The listing builds one solid part. Answer for the finished solid, in the listing's coordinates (mm). Give positions to 0.01 mm unless a question says otherwise; leave off trailing zeros. Write each loop counter-clockwise with the first axis right and the second up, starting at its lowest first coordinate (ties: lowest second). Pieces come first, ordered by that corner, then holes. Notation, with made-up numbers: M 71.5,-16 L 118.5,-16 A11 cw 118.5,3 Z; hole C -31.5,30.5 d11. An arc over 180 degrees is marked long. Answer as a JSON object with one key per item and string values.
```python
from build123d import *

# Parameters (mm, degrees)
SKETCH_1_R          = 1.5
SKETCH_1_W          = 4
SKETCH_1_H          = 35
EXTRUDE_1_DEPTH     = 3
FILLET_1_R          = 2
SKETCH_2_R          = 11
CUT_EXTRUDE_1_DEPTH = 3


with BuildPart() as part:
    # 草图1 → 凸台-拉伸1 (new body)
    with BuildSketch(Plane.XY):
        Polygon((-20, 25), (-25, 20), (-25, -75), (-20, -80), (20, -80), (25, -75), (25, 20), (20, 25), align=None)
        with Locations((-15.5, 15.5)):
            Circle(SKETCH_1_R, mode=Mode.SUBTRACT)
        with Locations((15.5, 15.5)):
            Circle(SKETCH_1_R, mode=Mode.SUBTRACT)
        with Locations((15.5, -15.5)):
            Circle(SKETCH_1_R, mode=Mode.SUBTRACT)
        with Locations((-15.5, -15.5)):
            Circle(SKETCH_1_R, mode=Mode.SUBTRACT)
        with Locations((-15.5, -55)):
            Rectangle(SKETCH_1_W, SKETCH_1_H, mode=Mode.SUBTRACT)
        with Locations((15.5, -55)):
            Rectangle(SKETCH_1_W, SKETCH_1_H, mode=Mode.SUBTRACT)
    extrude(amount=EXTRUDE_1_DEPTH)

    # 圆角1
    fillet_1_edges = [part.edges().sort_by_distance(p)[0] for p in [
        (17.5, -72.5, 1.5),
        (-13.5, -72.5, 1.5),
        (13.5, -37.5, 1.5),
        (-17.5, -37.5, 1.5),
        (-17.5, -72.5, 1.5),
        (13.5, -72.5, 1.5),
        (17.5, -37.5, 1.5),
        (-13.5, -37.5, 1.5),
    ]]
    fillet(fillet_1_edges, radius=FILLET_1_R - 0.0001)  # a hair under: the kernel refuses the full size

    # 草图2 → 切除-拉伸1 (cut)
    with BuildSketch(Plane.XY.offset(3)):
        Circle(SKETCH_2_R)
    extrude(amount=-CUT_EXTRUDE_1_DEPTH, mode=Mode.SUBTRACT)


solid = part.part
```
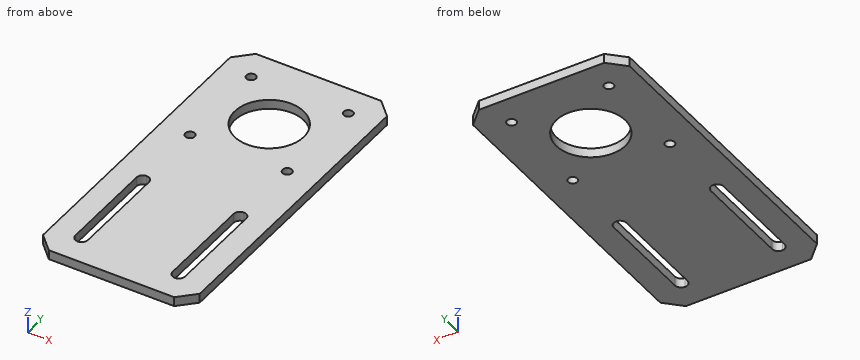
1. A cutting plane is placed at B-B, the plane y = 0. Give the vertices of the cut face in (x, z), plus the area to 3 significant figures.
Verdict:
{"outline": "M -25,0 L -11,0 L -11,3 L -25,3 Z; M 11,0 L 25,0 L 25,3 L 11,3 Z", "area": "84.0 mm2"}
2. A cutting plane is placed at D-D, the plane y = 15.5. Give the vertices of the cut face in (x, z), plus the area to 3 significant figures.
Verdict:
{"outline": "M -25,0 L -17,0 L -17,3 L -25,3 Z; M -14,0 L 14,0 L 14,3 L -14,3 Z; M 17,0 L 25,0 L 25,3 L 17,3 Z", "area": "132 mm2"}
3. A cutting plane is placed at C-C, the plane z = 1.8. Count the separate pieces of the cut face and the enclosed holes in it, plus the area to 3 significant figures.
Verdict:
{"separate pieces": "1", "enclosed holes": "7", "area": "4,520 mm2"}
4. A flat-ended cylindrical pin translates along its axis: pin 1 (5 mm diameter, centred on x = 15.5, y = -15.5, fed in from -Z). Find the tip coordinate at first contact, or state that the pin passes through.
Verdict:
{"pin 1": "stops at z = 0"}
5. A cutting plane is placed at A-A, the plane x = 0. Give the vertices of the cut face in (y, z).
Verdict:
{"outline": "M -80,0 L -11,0 L -11,3 L -80,3 Z; M 11,0 L 25,0 L 25,3 L 11,3 Z"}
6. Consider line 1 along X through (y, z) = (-53, 2.35); line 2 along Y through (x, z) = (-15.5, 2); line 3 along Y through (x, z) = (0, 2). Determine where each line is inside the solid, lowest interval first.
Verdict:
{"line 1": "x = -25 to -17.5, -13.5 to 13.5, 17.5 to 25", "line 2": "y = -80 to -72.5, -37.5 to -17, -14 to 14, 17 to 25", "line 3": "y = -80 to -11, 11 to 25"}
